Source: CAD feature listing. Evaluate the final solid. Frame: model axes, mm. A direction names the side the tool comes from. Give positions to 0.01 mm unless a question says otherwise; leave off trailing zeros. Order: outer loops, then holes, each group sorted by start corner. A loop starts at its lowest first (then second) coordinate and runs counter-clockwise, first axis right, second up. Notation, with made-up numbers: M 54.5,-3 L 75.5,-3 A29 cw 75.5,32 Z; hole C -9,41.5 d9. An arc over 180 degrees is marked long. Answer as a JSON object with one key per item and string values. Group by question number.
1. Section query D-D (y = 36). Output: boundary loops of the cut face in (x, z).
2. Pin query (flat end, axial travel): P1, Ø1.5, axis at x = 41.5, z = -50, coming from the -Y side; P2, Ø1, axis at x = 71.5, z = -80.5, coming from the +Y side. Return the tip coordinate at first contact, or that it passes through.
3. Section query B-B (x = 22.5). Output: boundary loops of the cut face in (y, z), plus the area to 4 significant figures.
4. Pull-direction query (Z, two-part tool) for faces 4 (the cylindrical face through (19.248, 55.357, -92.395)), 5 (the flat face through (100, 10, -30)), 6 (the flat face through (50, 37, -100)); classes: +Z half, -Z half, draft (parallel to the pull), parting line (faces both ways), or undercut.
5. Set-up query: faces 1 (the flat face through (99, 10, -70)), 2 (the flat face through (61.078, 50.498, -7.395)), 3 (the flat face through (31, 48, -15)). Return all of +Z, -Z, +X, -X, +Y, -Y with unobstructed straight access to the full face (end or side cutting, diameter ignored); none if empty.
6. Section query C-C (y = 14.5). Output: boundary loops of the cut face in (x, z), plus the area to 3 significant figures.
7. Section query A-A (z = -92). Output: boundary loops of the cut face in (x, y), plus the area to 3 significant figures.
8. Material intervals for L1, parallel to Y at x = 22, z = -4; L2, parallel to Z at x = 51, y = 42.5; L3, parallel to Y at x = 38.5, z = -52, sorted ascending. Write a range as [from, to].
from build123d import *

# Parameters (mm, degrees)
SKETCH1_R           = 22.5
SKETCH1_R_2         = 15
BOSS_EXTRUDE1_DEPTH = 100
SKETCH2_W           = 167.207150193
SKETCH2_H           = 70
CUT_EXTRUDE1_DEPTH  = 73.5
CUT_EXTRUDE2_DEPTH  = 21


with BuildPart() as part:
    # Sketch1 → Boss-Extrude1 (new body)
    with BuildSketch(Plane.XY):
        with BuildLine():
            Line((0, 70), (0, 0))
            Line((0, 0), (130, 0))
            Line((130, 0), (110, 20))
            Line((110, 20), (80, 20))
            Line((80, 20), (41.61915802, 81.862031723))
            ThreePointArc((41.61915802, 81.862031723), (44.138288466, 76.16720944), (45, 70))
            ThreePointArc((45, 70), (22.5, 47.5), (0, 70))
        make_face()
        with Locations((22.5, 70)):
            Circle(SKETCH1_R)
        with Locations((22.5, 70)):
            Circle(SKETCH1_R_2, mode=Mode.SUBTRACT)
    extrude(amount=-BOSS_EXTRUDE1_DEPTH)

    # Sketch2 → Cut-Extrude1 (cut, through all)
    with BuildSketch(Plane(origin=(0, 20, 0), x_dir=(1, 0, 0), z_dir=(0, 1, 0))):
        with Locations((64.505889037, 50)):
            Rectangle(SKETCH2_W, SKETCH2_H)
    extrude(amount=CUT_EXTRUDE1_DEPTH, mode=Mode.SUBTRACT)

    # Sketch3 → Cut-Extrude2 (cut, through all)
    with BuildSketch(Plane(origin=(0, 20, 0), x_dir=(1, 0, 0), z_dir=(0, 1, 0))):
        with BuildLine():
            Line((80, 70), (130, 70))
            Line((130, 70), (130, 30))
            Line((130, 30), (80, 30))
            ThreePointArc((80, 30), (60, 50), (80, 70))
        make_face()
    extrude(amount=-CUT_EXTRUDE2_DEPTH, mode=Mode.SUBTRACT)


solid = part.part
Answer sheet:
{
 "1": {"outline": "M 0,-100 L 70.07,-100 L 70.07,-85 L 0,-85 Z; M 0,-15 L 70.07,-15 L 70.07,0 L 0,0 Z"},
 "2": {"P1": "y = 0", "P2": "y = 20"},
 "3": {"outline": "M 0,-100 L 55,-100 L 55,-85 L 20,-85 L 20,-15 L 55,-15 L 55,0 L 0,0 Z; M 85,-100 L 92.5,-100 L 92.5,-85 L 85,-85 Z; M 85,-15 L 92.5,-15 L 92.5,0 L 85,0 Z", "area": "3,275 mm^2"},
 "4": {"face 4": "draft", "face 5": "undercut", "face 6": "-Z half"},
 "5": {"face 1": "+X, +Y, -Y", "face 2": "+Z, -Z, +X, +Y", "face 3": "+X, -X, +Y"},
 "6": {"outline": "M 0,-100 L 115.5,-100 L 115.5,-70 L 80,-70 A20 cw 80,-30 L 115.5,-30 L 115.5,0 L 0,0 Z", "area": "9,500 mm^2"},
 "7": {"outline": "M 0,0 L 130,0 L 110,20 L 80,20 L 41.62,81.86 A22.5 ccw 0,70 Z; hole C 22.5,70 d30", "area": "5,730 mm^2"},
 "8": {"L1": "[0, 55.01], [84.99, 92.49]", "L2": "[-100, -85], [-15, 0]", "L3": "[0, 20]"}
}
